Geometry check sheet. Reference: the model listing, model coordinates, mm. Face numbers are marked on the shaded views. A direction names the side the tool comes from. Coordinates: 2 decimals unless noted, no trailing zeros. Write each loop counter-clockwise with the first axis right and the second up, starting at its lowest first coordinate (ties: lowest second). Pieces come first, ordered by that corner, then holes. Notation, with made-up numbers: (36, -23) -> (59, -23) arc R21 cw to (59, -12) -> close; hole circle Ø2 at (84, 74.25). An arc over 180 degrees is marked (long way). Use a Markdown table: item, result.
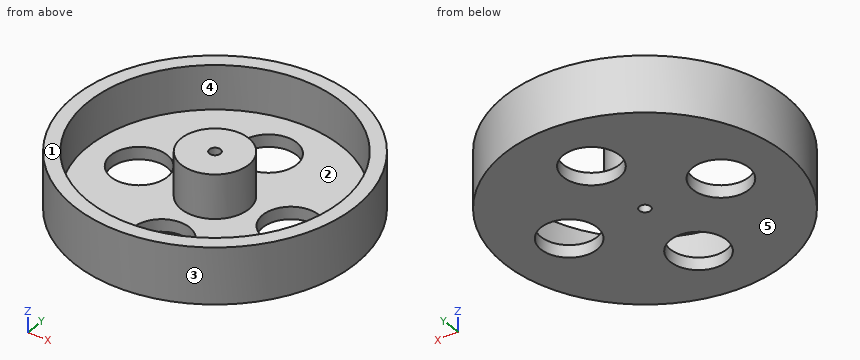
```python
from build123d import *

# Parameters (mm, degrees)
SKETCH1_R                 = 25
WHEEL_WEB_50MM_DEPTH      = 2.2
OUTER_RIM_10MM_WIDE_START = 2.2
SKETCH2_R                 = 25
SKETCH2_R_2               = 22.5
OUTER_RIM_10MM_WIDE_DEPTH = 7.8
HUB_12MM_START            = 2.2
SKETCH3_R                 = 6
HUB_12MM_DEPTH            = 7.8
AXLE_BORE_FIT_CHECK_START = -0.1
SKETCH4_R                 = 1
AXLE_BORE_FIT_CHECK_DEPTH = 10.2
LIGHTENING_X_13_5_START   = -0.1
SKETCH5_R                 = 5
LIGHTENING_X_13_5_DEPTH   = 10.2
SKETCH6_R                 = 5
LIGHTENING_X_13_5_2_DEPTH = 10.2
LIGHTENING_Y_13_5_START   = -0.1
SKETCH7_R                 = 5
LIGHTENING_Y_13_5_DEPTH   = 10.2
SKETCH8_R                 = 5
LIGHTENING_Y_13_5_2_DEPTH = 10.2


with BuildPart() as part:
    # Sketch1 → Wheel_Web_50mm (new body)
    with BuildSketch(Plane.XY):
        Circle(SKETCH1_R)
    extrude(amount=WHEEL_WEB_50MM_DEPTH)

    # Sketch2 → Outer_Rim_10mm_Wide (add)
    with BuildSketch(Plane.XY.offset(OUTER_RIM_10MM_WIDE_START)):
        Circle(SKETCH2_R)
        Circle(SKETCH2_R_2, mode=Mode.SUBTRACT)
    extrude(amount=OUTER_RIM_10MM_WIDE_DEPTH)

    # Sketch3 → Hub_12mm (add)
    with BuildSketch(Plane.XY.offset(HUB_12MM_START)):
        Circle(SKETCH3_R)
    extrude(amount=HUB_12MM_DEPTH)

    # Sketch4 → Axle_Bore_FIT_CHECK (cut)
    with BuildSketch(Plane.XY.offset(AXLE_BORE_FIT_CHECK_START)):
        Circle(SKETCH4_R)
    extrude(amount=AXLE_BORE_FIT_CHECK_DEPTH, mode=Mode.SUBTRACT)

    # Sketch5 → Lightening_X_-13.5 (cut)
    with BuildSketch(Plane.XY.offset(LIGHTENING_X_13_5_START)):
        with Locations((-13.5, 0)):
            Circle(SKETCH5_R)
    extrude(amount=LIGHTENING_X_13_5_DEPTH, mode=Mode.SUBTRACT)

    # Sketch6 → Lightening_X_13.5 2 (cut)
    with BuildSketch(Plane.XY.offset(LIGHTENING_X_13_5_START)):
        with Locations((13.5, 0)):
            Circle(SKETCH6_R)
    extrude(amount=LIGHTENING_X_13_5_2_DEPTH, mode=Mode.SUBTRACT)

    # Sketch7 → Lightening_Y_-13.5 (cut)
    with BuildSketch(Plane.XY.offset(LIGHTENING_Y_13_5_START)):
        with Locations((0, -13.5)):
            Circle(SKETCH7_R)
    extrude(amount=LIGHTENING_Y_13_5_DEPTH, mode=Mode.SUBTRACT)

    # Sketch8 → Lightening_Y_13.5 2 (cut)
    with BuildSketch(Plane.XY.offset(LIGHTENING_Y_13_5_START)):
        with Locations((0, 13.5)):
            Circle(SKETCH8_R)
    extrude(amount=LIGHTENING_Y_13_5_2_DEPTH, mode=Mode.SUBTRACT)


solid = part.part
```
Item 1: Depth check by flat-ended pin: P1, Ø4, axis at x = -7.5, z = 8.5, coming from the +Y side; P2, Ø1, axis at y = -18.5, z = 5.5, coming from the -X side; P3, Ø4, axis at y = -16, z = 5.5, coming from the +X side; P4, Ø8, axis at x = 0, y = -13.5, coming from the -Z side. Enter the tip coordinate at first touch or a pass-through.
Answer block:
| item | result |
|---|---|
| P1 | stops at y = 24.39 |
| P2 | stops at x = -17.35 |
| P3 | stops at x = 20.71 |
| P4 | passes through |
Item 2: Thickness scan on L1, parallel to Y at x = 0, z = 8; L2, parallel to X at y = 5.5, z = 8.5; L3, parallel to X at y = -2.5, z = 5.25. Record the ranges inside material, lowest first. Write a range as [from, to].
Answer block:
| item | result |
|---|---|
| L1 | y = [-25, -22.5], [-6, -1], [1, 6], [22.5, 25] |
| L2 | x = [-24.39, -21.82], [-2.4, 2.4], [21.82, 24.39] |
| L3 | x = [-24.87, -22.36], [-5.45, 5.45], [22.36, 24.87] |
Item 3: Mould release check, pull along Y, two halves, no side actions. Record for the marked faces 3, 4 and 5: +Y half, -Y half, draft (parallel to the pull), parting line (faces both ways), or undercut.
Answer block:
| item | result |
|---|---|
| face 3 | parting line |
| face 4 | undercut |
| face 5 | draft |
Item 4: Section check C-C on x = -4. Record the boundary of the cut face in (y, z).
Answer block:
| item | result |
|---|---|
| outline | (-24.68, 0) -> (-16.5, 0) -> (-16.5, 2.2) -> (-22.14, 2.2) -> (-22.14, 10) -> (-24.68, 10) -> close; (-10.5, 0) -> (10.5, 0) -> (10.5, 2.2) -> (4.47, 2.2) -> (4.47, 10) -> (-4.47, 10) -> (-4.47, 2.2) -> (-10.5, 2.2) -> close; (16.5, 0) -> (24.68, 0) -> (24.68, 10) -> (22.14, 10) -> (22.14, 2.2) -> (16.5, 2.2) -> close |
Item 5: Section check D-D on y = -11. Record the boundary of the cut face in (x, z).
Answer block:
| item | result |
|---|---|
| outline | (-22.45, 0) -> (-4.33, 0) -> (-4.33, 2.2) -> (-19.63, 2.2) -> (-19.63, 10) -> (-22.45, 10) -> close; (4.33, 0) -> (22.45, 0) -> (22.45, 10) -> (19.63, 10) -> (19.63, 2.2) -> (4.33, 2.2) -> close |
Item 6: Tool access check on the marked faces 1 and 2. Record the directions out of +Z, -Z, +X, -X, +Y, -Y that give a thin tool (end or side, any length) a straight path to the whole face; none if there is none.
Answer block:
| item | result |
|---|---|
| face 1 | +Z, +X, -X, +Y, -Y |
| face 2 | +Z |
Item 7: Section check B-B on y = 0. Record the boundary of the cut face in (x, z), then the cut area to 3 significant figures.
Answer block:
| item | result |
|---|---|
| outline | (-25, 0) -> (-18.5, 0) -> (-18.5, 2.2) -> (-22.5, 2.2) -> (-22.5, 10) -> (-25, 10) -> close; (-8.5, 0) -> (-1, 0) -> (-1, 10) -> (-6, 10) -> (-6, 2.2) -> (-8.5, 2.2) -> close; (1, 0) -> (8.5, 0) -> (8.5, 2.2) -> (6, 2.2) -> (6, 10) -> (1, 10) -> close; (18.5, 0) -> (25, 0) -> (25, 10) -> (22.5, 10) -> (22.5, 2.2) -> (18.5, 2.2) -> close |
| area | 179 mm^2 |
Item 8: Section check A-A on z = 5.5. Record the boundary of the cut face in (x, y), then the cut area to 3 significant figures.
Answer block:
| item | result |
|---|---|
| outline | circle Ø50 at (0, 0); circle Ø12 at (0, 0); hole circle Ø45 at (0, 0); hole circle Ø2 at (0, 0) |
| area | 483 mm^2 |
